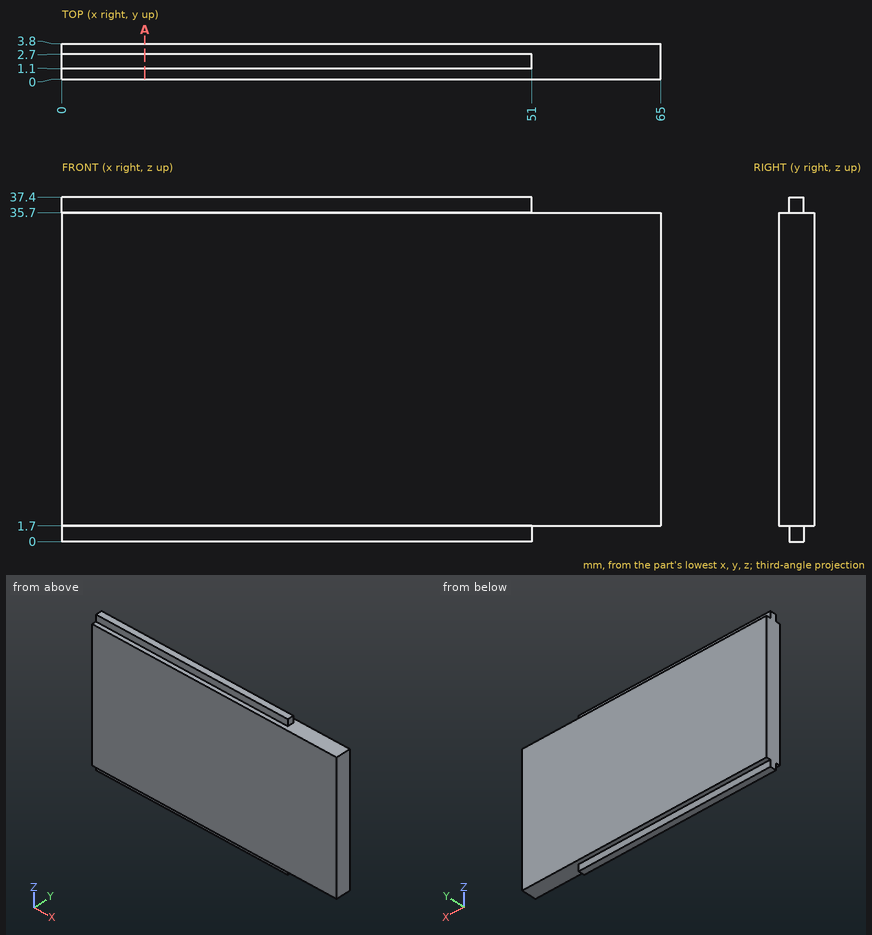
Verification items for this drawing (mm, ordinates from the low corner). Coordinates: 2 decimals unless noted, no trailing zeros. Write each loop counter-clockwise with the first axis right and the second up, starting at its lowest first coordinate (ties: lowest second). Pieces come first, ordered by that corner, then holes. Notation, with made-up numbers: (86, 13) -> (96, 13) arc R22 ccw to (96, 45) -> close; hole circle Ø5 at (68, 17). An arc over 180 degrees is marked (long way). One line per item, written item: value. Start each with the question number.
Q1. Cross-section at A-A on x = 9. Enter the section's corners in (y, z).
Q2. Thickness scan on L1, parallel to Z at x = 42.5, y = 0.75. Record the ranges inside material, lowest first. Write a range as from..to.
Q3. Go/stop test with flat-tipped pins: P1, Ø1.8, axis at y = 2, z = 0.5, coming from the +X side; P2, Ø1.4, axis at x = 16.5, z = 36.5, coming from the +Y side; P3, Ø1.9, axis at x = 26, z = 37, coming from the -Y side. Record where each tip stops, or that it passes through.
Checked values:
1. outline: (0, 1.7) -> (1.1, 1.7) -> (1.1, 0) -> (2.7, 0) -> (2.7, 1.7) -> (3.8, 1.7) -> (3.8, 35.7) -> (2.7, 35.7) -> (2.7, 37.4) -> (1.1, 37.4) -> (1.1, 35.7) -> (0, 35.7) -> close
2. L1: z = 1.7..35.7
3. P1: stops at x = 51
3. P2: stops at y = 2.7
3. P3: stops at y = 1.1
